For this review, take the finished solid that the model builds, in its own axes (mm). A direction names the side the tool comes from. Coordinates: 2 decimals unless noted, no trailing zeros. Write each loop counter-clockwise with the first axis right and the second up, starting at its lowest first coordinate (ties: lowest second). Pieces come first, ordered by that corner, then holes.
```python
from build123d import *

# Parameters (mm, degrees)
F0_W     = 1958
F0_H     = 1715
F1_DEPTH = 4
F2_W     = 582
F2_H     = 710
F3_DEPTH = 4.001
F5_DEPTH = 4.001
F6_R     = 90


with BuildPart() as f1:
    # F0 (on Right) → F1 (new body)
    with BuildSketch(Plane.YZ):
        Rectangle(F0_W, F0_H)
    extrude(amount=F1_DEPTH)

    # F2 (on face) → F3 (cut, through all)
    with BuildSketch(Plane.YZ.offset(4)):
        Polygon((697, 857.5), (979, -147.5), (979, 857.5), align=None)
        with Locations((688, -502.5)):
            Rectangle(F2_W, F2_H)
    extrude(amount=-F3_DEPTH, mode=Mode.SUBTRACT)

    # F4 (on face) → F5 (cut, through all)
    with BuildSketch(Plane.YZ.offset(4)):
        Polygon((353.608048, 797.5), (-206, 799.5), (-206, -52.5), (519.614009, -57.5), (519.614009, 7.5), align=None)
    extrude(amount=-F5_DEPTH, mode=Mode.SUBTRACT)

    # F6
    f6_edges = [f1.edges().sort_by_distance(p)[0] for p in [
        (2, -206, 799.5),
        (2, 353.608048, 797.5),
    ]]
    fillet(f6_edges, radius=F6_R)


solid = f1.part
```
1) Consider section A-A (z = 311). Give the boundary of the cut face in (x, y), then the cut area to 3 significant figures.
2) For L1, parallel to Z at x = 1.7, y = 556.5; L2, parallel to Y at x = 3.5, z = -495.5; L3, parallel to Z at x = 2.2, y = 246.5, list the stretches that pass through material, from the lowest coordinate up.
3) Tool access review of faces 1 (the face through (1.972, 336.678, 778.075)), 2 (the face through (4, -231, 12)): name each direction out of +Z, -Z, +X, -X, +Y, -Y from which nothing blocks a thin tool from reaching the whole face with its end or side.
4) Clearance check with flat-ended pins moving along their axes: P1, Ø1.2, axis at x = 2, z = -636.5, coming from the +Y side; P2, Ø8, axis at y = -130.5, z = -334.5, coming from the -X side; P3, Ø1, axis at x = 0.5, z = -57, coming from the +Y side. State where each tip first meets the part, or that it passes through.
5) The part is to be moulded in two halves that separate along Y. For faces 3 (the face through (0, -231, 12)), 4 (the face through (2.028, 836.026, 362.035)), 5 (the face through (2.028, 445.152, 361.853)), say which applies: pulls with the +Y half, pulls with the -Y half, needs draft (parallel to the pull), parting line crosses it, or undercut.
6) Consider section B-B (x = 0.8). Give the boundary of the cut face in (y, z).
7) Consider section C-C (z = -476). Give the boundary of the cut face in (x, y).
8) Consider section D-D (z = 581). Give the boundary of the cut face in (x, y).
Results:
1. outline: (0, -979) - (4, -979) - (4, -206) - (0, -206) - close; (0, 455.84) - (4, 455.84) - (4, 850.35) - (0, 850.35) - close
1. area: 4,670 mm2
2. L1: z = -147.5 to 857.5
2. L2: y = -979 to 397
2. L3: z = -857.5 to -55.62, 797.88 to 857.5
3. face 1: +X, -X
3. face 2: +Z, -Z, +X, +Y, -Y
4. P1: stops at y = 397
4. P2: stops at x = 0
4. P3: stops at y = 953.75
5. face 3: needs draft
5. face 4: pulls with the +Y half
5. face 5: undercut
6. outline: (-979, -857.5) - (397, -857.5) - (397, -147.5) - (979, -147.5) - (697, 857.5) - (-979, 857.5) - close; hole (-206, -52.5) - (519.61, -57.5) - (519.61, 7.5) - (368.58, 726.27) arc R90 ccw to (280.82, 797.76) - (-115.68, 799.18) arc R90 ccw to (-206, 709.18) - close
7. outline: (0, -979) - (4, -979) - (4, 397) - (0, 397) - close
8. outline: (0, -979) - (4, -979) - (4, -206) - (0, -206) - close; (0, 399.1) - (4, 399.1) - (4, 774.59) - (0, 774.59) - close
